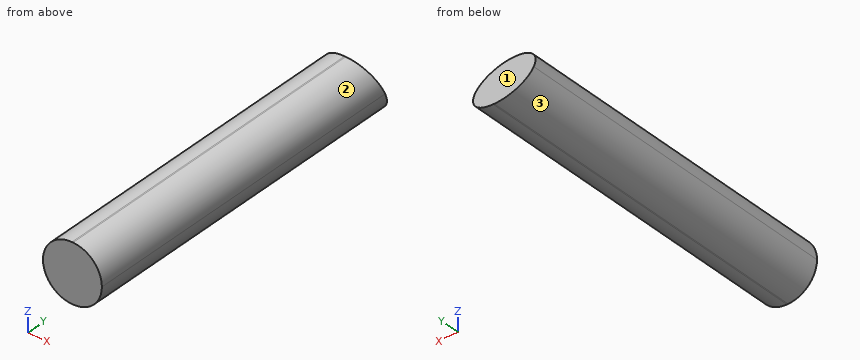
from build123d import *

# Parameters (mm, degrees)
F2_DEPTH = 12.954
F3_R     = 6.34999


# Not quite as in the source:
# - a fillet or chamfer is up to 0.001 mm smaller than in the source, because OpenCascade refuses the exact size


with BuildPart() as f2:
    # F1 (on Right) → F2 (new body)
    with BuildSketch(Plane.YZ):
        Polygon((-39.228890075, 12.7), (-39.228890075, 0), (39.228890075, 0), (33.5844452765, 12.7), align=None)
    extrude(amount=F2_DEPTH)

    # F3 (radius 6.35 in the source; OpenCascade refuses exactly that, so slightly less here)
    f3_edges = [f2.edges().sort_by_distance(p)[0] for p in [
        (12.954, 0, 0),
        (12.954, -2.822222, 12.7),
        (0, -2.822222, 12.7),
        (0, 0, 0),
    ]]
    fillet(f3_edges, radius=F3_R)


solid = f2.part
Part model, mm, in its own coordinate system. Face numbers are marked on the shaded views. Give positions to 0.01 mm unless a question says otherwise; leave off trailing zeros. Loops run counter-clockwise (first coordinate to the right, second up) from the corner with the lowest first, then second, coordinate; pieces in that order, holes last. Notation, with made-up numbers: (17.5, 62.5) -> (23.5, 62.5) arc R13 cw to (23.5, 79.5) -> close; hole circle Ø7 at (52, 65). An arc over 180 degrees is marked (long way). Write each question's results on one line, items separated by ' | '. Start each with the question number.
Q1. Wall check: L1, parallel to X at y = -11, z = 6; L2, parallel to Z at x = 7, y = 19.5; L3, parallel to Y at x = 9.5, z = 4. Give the ranges that are in metal, low to high.
Q2. Band-saw the part on B-B on z = 5. List the corners of the cut face in (x, y), plus the area to 3 significant figures.
Q3. Pin check, flat tips, straight feed: P1, Ø2, axis at y = -10, z = 3.5, coming from the +X side; P2, Ø1, axis at y = 31, z = 1.5, coming from the -X side; P3, Ø1, axis at x = 3.5, y = 1, coming from the +Z side. Stop position of each tip, or through.
Q4. Band-saw the part on C-C on x = 2.75. List the corners of the cut face in (y, z), plus the area to 3 significant figures.
Q5. Pull direction X, two halves, no side cores. Call the marked faces 1, 2 and 3: +X half, -X half, draft (parallel to the pull), parting line (faces both ways), or undercut.
Results are:
1) L1: x = 0.01 to 12.94 | L2: z = 0.01 to 12.69 | L3: y = -39.23 to 37.45
2) outline: (0.15, -39.23) -> (12.81, -39.23) -> (12.81, 37.01) -> (0.15, 37.01) -> close | area: 965 mm²
3) P1: stops at x = 12.68 | P2: stops at x = 1.72 | P3: stops at z = 12.25
4) outline: (-39.23, 1.12) -> (38.73, 1.12) -> (34.08, 11.58) -> (-39.23, 11.58) -> close | area: 791 mm²
5) face 1: draft | face 2: +X half | face 3: -X half
